Geometry check sheet. Reference: the model listing, model coordinates, mm. A direction names the side the tool comes from. Round coordinates to 2 decimals unless told otherwise and drop trailing zeros. Loops run counter-clockwise (first coordinate to the right, second up) from the corner with the lowest first, then second, coordinate; pieces in that order, holes last. Notation, with made-up numbers: (45.5, 78.25) -> (58.5, 78.25) arc R8 cw to (58.5, 86.25) -> close; hole circle Ø1 at (42.5, 18). An arc over 180 degrees is marked (long way). Use a Markdown table: item, result. Add a question column.
Q1. Material ranges on L1, parallel to Y at x = 30, z = 80.5; L2, parallel to Y at x = 77.5, z = 50.5; L3, parallel to Z at x = -91.5, y = 4.25, recorded low to high.
Q2. Set-up check for faces 1 (the face through (-2, 15, -117)), 2 (the face through (-2.065, 21.744, -93.299)), 3 (the face through (-2.037, 22.238, 54.186)): record each of +Z, -Z, +X, -X, +Y, -Y from which the full face is reachable in a straight line by a thin tool's end or side.
Q3. Sectioned sample at A-A, the plane x = -129. Enter the section's corners in (y, z).
Q4. Release check for a two-part mould opening along X. For faces 4 (the face through (147.5, 16, 2)), 5 (the face through (-2, 16, 117)), 6 (the face through (-2, 21.031, 72)), 7 (the face through (145.5, 24, 72)) record: released by +X, released by -X, zero draft, split by the parting line, or undercut.
Q5. Sectioned sample at C-C, the plane z = -64. Enter the section's corners in (x, y).
Q6. Sectioned sample at B-B, the plane z = 1. Enter the section's corners in (x, y).
Q7. Gauge pin test, flat ends, axial feed: P1, Ø22.5, axis at x = -22, z = 78.5, coming from the +Y side; P2, Ø10, axis at x = 51, z = 84.5, coming from the +Y side; P3, Ø2, axis at x = 4, z = -116, coming from the +Y side. Record the tip position at first contact, or that the pin passes through.
```python
from build123d import *

# Parameters (mm, degrees)
SKETCH1_W           = 295
SKETCH1_H           = 234
BOSS_EXTRUDE1_DEPTH = 28
CUT_EXTRUDE1_DEPTH  = 300
CHAMFER1_SIZE       = 5
CHAMFER2_SIZE       = 5
SKETCH3_W           = 40
SKETCH3_H           = 12.256911823
CUT_EXTRUDE2_DEPTH  = 300
BOSS_EXTRUDE2_DEPTH = 2
BOSS_EXTRUDE3_DEPTH = 295
FILLET1_R           = 6
FILLET2_R           = 6
CHAMFER3_SIZE       = 5


with BuildPart() as part:
    # Sketch1 → Boss-Extrude1 (new body)
    with BuildSketch(Plane(origin=(0, 0, 0), x_dir=(1, 0, 0), z_dir=(0, 1, 0))):
        Rectangle(SKETCH1_W, SKETCH1_H)
    extrude(amount=BOSS_EXTRUDE1_DEPTH)

    # Sketch2 → Cut-Extrude1 (cut)
    with BuildSketch(Plane.ZY.offset(147.5)):
        Polygon((117, 28), (-76.5, 20.5), (-117, 23.5), (-117, 28), align=None)
    extrude(amount=-CUT_EXTRUDE1_DEPTH, mode=Mode.SUBTRACT)

    # Chamfer1
    chamfer1_edges = [part.edges().sort_by_distance(p)[0] for p in [
        (147.5, 0, 0),
        (-147.5, 0, 0),
    ]]
    chamfer(chamfer1_edges, length=CHAMFER1_SIZE)

    # Chamfer2
    chamfer2_edges = [part.edges().sort_by_distance(p)[0] for p in [
        (0, 0, 117),
    ]]
    chamfer(chamfer2_edges, length=CHAMFER2_SIZE)

    # Sketch3 → Cut-Extrude2 (cut)
    with BuildSketch(Plane.ZY.offset(147.5)):
        with Locations((72, 27.159463664)):
            Rectangle(SKETCH3_W, SKETCH3_H)
    extrude(amount=-CUT_EXTRUDE2_DEPTH, mode=Mode.SUBTRACT)

    # Sketch4 → Boss-Extrude2 (add)
    with BuildSketch(Plane.ZY.offset(147.5)):
        Polygon((92, 27.031007752), (52, 25.480620155), (52, 21.031007752), (92, 21.031007752), align=None)
    boss_extrude2 = extrude(amount=-BOSS_EXTRUDE2_DEPTH)

    # Mirror1: Boss-Extrude2 across plane
    add(boss_extrude2.mirror(Plane(origin=(0, 0, 0), x_dir=(0, 0, 1), z_dir=(1, 0, 0))))

    # Sketch5 → Boss-Extrude3 (add)
    with BuildSketch(Plane.ZY.offset(147.5)):
        Polygon((-117, 23.5), (-115, 23.351851852), (-115, 25.5), (-117, 25.5), align=None)
    extrude(amount=-BOSS_EXTRUDE3_DEPTH)

    # Fillet1
    # the kernel refuses this fillet: 6 mm, written as the material it adds along each edge
    with BuildSketch(Plane(origin=(-147.5, 23.351851852, -115), x_dir=(0, -0.0738716855153118, 0.997267754456709), z_dir=(1, 0, 0))) as fillet1_piece_1:
        with BuildLine():
            CenterArc((4.436743859, -6), FILLET1_R, 90, 49.987589721)
            Line((-0.158687324, -2.14227888), (-0.250595948, -2.065124458))
            ThreePointArc((-0.250595948, -2.065124458), (-0.199015793, -1.062274838), (-0.119672131, 0.008864602))
            Line((-0.119672131, 0.008864602), (0, 0.12))
            Line((0, 0.12), (4.436743859, 0.12))
            Line((4.436743859, 0.12), (4.436743859, 0))
        make_face()
    extrude(amount=295)

    # Fillet2
    # the kernel refuses this fillet: 6 mm, written as the material it adds along each edge
    with BuildSketch(Plane(origin=(-145.5, 21.031007752, 92), x_dir=(0, 1, 0), z_dir=(1, 0, 0))) as fillet2_piece_1:
        with BuildLine():
            CenterArc((FILLET2_R, -FILLET2_R), FILLET2_R, 90, 90)
            Line((0, -FILLET2_R), (-FILLET2_R * 0.02, -FILLET2_R))
            Line((-FILLET2_R * 0.02, -FILLET2_R), (-FILLET2_R * 0.02, FILLET2_R * 0.02))
            Line((-FILLET2_R * 0.02, FILLET2_R * 0.02), (FILLET2_R, FILLET2_R * 0.02))
            Line((FILLET2_R, FILLET2_R * 0.02), (FILLET2_R, 0))
        make_face()
    extrude(amount=291)
    with BuildSketch(Plane(origin=(-145.5, 21.031007752, 52), x_dir=(0, 1, 0), z_dir=(1, 0, 0))) as fillet2_piece_2:
        with BuildLine():
            CenterArc((6, 5.796231388), FILLET2_R, 180, 75.024977641)
            Line((0, 5.796231388), (-0.12, 5.796231388))
            Line((-0.12, 5.796231388), (-0.12, 0))
            Line((-0.12, 0), (0, -0.12))
            ThreePointArc((0, -0.12), (2.224806202, -0.12), (4.418604651, -0.115924628))
            Line((4.418604651, -0.115924628), (4.449612403, 0))
        make_face()
    extrude(amount=291)

    # Chamfer3
    chamfer3_edges = [part.edges().sort_by_distance(p)[0] for p in [
        (0, 0, -117),
    ]]
    chamfer(chamfer3_edges, length=CHAMFER3_SIZE)


solid = part.part
```
Values:
| question | item | result |
|---|---|---|
| 1 | L1 | 0 to 21.03 |
| 1 | L2 | 0 to 25.42 |
| 1 | L3 | -116.25 to 116.25 |
| 2 | face 1 | -Z, +X, -X, +Y, -Y |
| 2 | face 2 | +X, -X, +Y |
| 2 | face 3 | +Y |
| 3 | outline | (0, -112) -> (5, -117) -> (25.5, -117) -> (25.5, -115) arc R6 cw to (23.02, -110.58) -> (20.5, -76.5) -> (25.48, 52) arc R6 cw to (21.03, 57.8) -> (21.03, 86) arc R6 cw to (27.03, 92) -> (28, 117) -> (5, 117) -> (0, 112) -> close |
| 4 | face 4 | released by +X |
| 4 | face 5 | zero draft |
| 4 | face 6 | undercut |
| 4 | face 7 | undercut |
| 5 | outline | (-147.5, 5) -> (-142.5, 0) -> (142.5, 0) -> (147.5, 5) -> (147.5, 20.98) -> (-147.5, 20.98) -> close |
| 6 | outline | (-147.5, 5) -> (-142.5, 0) -> (142.5, 0) -> (147.5, 5) -> (147.5, 23.5) -> (-147.5, 23.5) -> close |
| 7 | P1 | y = 22.35 |
| 7 | P2 | y = 22.16 |
| 7 | P3 | y = 25.5 |
